Model file for the job. Use its own axes, mm. Face numbers are marked on the shaded views. A direction names the side the tool comes from. Coordinates: 2 decimals unless noted, no trailing zeros. Order: outer loops, then holes, each group sorted by start corner. A loop starts at its lowest first (then second) coordinate and runs counter-clockwise, first axis right, second up.
from build123d import *

# Parameters (mm, degrees)
SKETCH_1_R          = 3
EXTRUDE_2_DEPTH     = 50
EXTRUDE_3_DEPTH     = 8
CUT_EXTRUDE_1_DEPTH = 26
SKETCH_3_R          = 4.5
EXTRUDE_4_DEPTH     = 1


with BuildPart() as part:
    # Sketch 1 → Extrude 2 (new body)
    with BuildSketch(Plane(origin=(0, 0, 0), x_dir=(1, 0, 0), z_dir=(0, 1, 0))):
        with Locations(Location((0, 0, 0), (0, 0, 270))):
            Circle(SKETCH_1_R)
    extrude(amount=EXTRUDE_2_DEPTH)

    # Sketch 1_3 → Extrude 3 (add)
    with BuildSketch(Plane(origin=(0, 0, 0), x_dir=(1, 0, 0), z_dir=(0, 1, 0))):
        with BuildLine():
            Line((-1, 4), (-1, 2.828427125))
            ThreePointArc((-1, 2.828427125), (0, 3), (1, 2.828427125))
            Line((1, 2.828427125), (1, 4))
            Line((1, 4), (-1, 4))
        make_face()
    extrude(amount=EXTRUDE_3_DEPTH)

    # Sketch 2 → Cut-Extrude 1 (cut)
    with BuildSketch(Plane(origin=(0, 50, 0), x_dir=(1, 0, 0), z_dir=(0, 1, 0))):
        Polygon((-1.2, 1.149545417), (1.2, 1.149545417), (1.2, 2.749545417), (0, 4.828006386), (-1.2, 2.749545417), align=None)
    extrude(amount=-CUT_EXTRUDE_1_DEPTH, mode=Mode.SUBTRACT)

    # Sketch 3 → Extrude 4 (add)
    with BuildSketch(Plane.XZ):
        with Locations(Location((0, 0, 0), (0, 0, 270))):
            Circle(SKETCH_3_R)
    extrude(amount=EXTRUDE_4_DEPTH)


solid = part.part
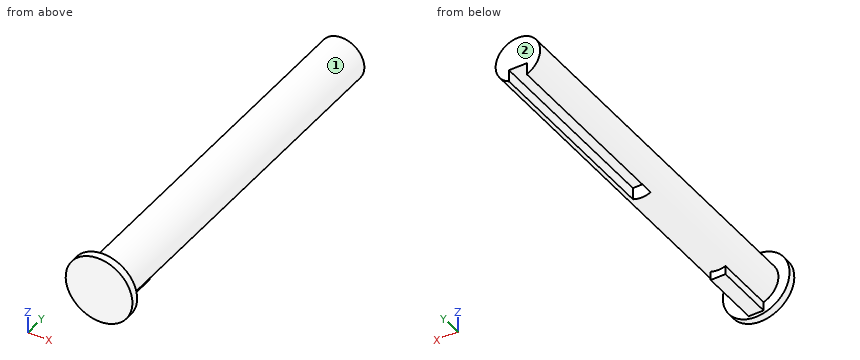
Q1. Probe line 1 (Y direction, x = 2.25, z = 3.5); line 2 (X direction, y = 4.5, z = -2.75); line 3 (Z direction, x = 0.25, y = 34.5). List the from-to ranges inside material, lowest first.
Established:
line 1: y = -1 to 0
line 2: x = -1.2 to 1.2
line 3: z = -1.15 to 2.99
Q2. Cut at B-B, the plane x = -1.75. List the corners of the cut face in (y, z).
Established:
outline: (-1, -4.15) - (0, -4.15) - (0, -2.44) - (50, -2.44) - (50, 2.44) - (0, 2.44) - (0, 4.15) - (-1, 4.15) - close
Q3. Cut at D-D, the plane z = -2. List the corners of the cut face in (x, y), plus the area to 3 significant figures.
Established:
outline: (-4.03, -1) - (4.03, -1) - (4.03, 0) - (2.24, 0) - (2.24, 50) - (1.2, 50) - (1.2, 24) - (-1.2, 24) - (-1.2, 50) - (-2.24, 50) - (-2.24, 0) - (-4.03, 0) - close
area: 169 mm2
Q4. Cut at A-A, the plane z = 0. List the corners of the cut face in (x, y), plus the area to 3 significant figures.
Established:
outline: (-4.5, -1) - (4.5, -1) - (4.5, 0) - (3, 0) - (3, 50) - (-3, 50) - (-3, 0) - (-4.5, 0) - close
area: 309 mm2
Q5. Cut at C-C, the plane y = 45.5. List the corners of the cut face in (x, z), plus the area to 3 significant figures.
Established:
outline: (-1.2, -2.75) - (-1.2, -1.15) - (1.2, -1.15) - (1.2, -2.75) arc R3 ccw (long way) to start
area: 24.0 mm2
Q6. Which spindle directions (+Z, -Z, +X, -X, +Y, -Y) get a long thin tool onto all of the face, cutting with end or side? Do the marked faces 1 and 2. Say none if no direction does.
Established:
face 1: +Y
face 2: +Z, -Z, +X, -X, +Y
Q7. Drop flat-ended pins along their axis: P1, Ø1.3, axis at y = 41.5, z = -1.5, coming from the +X side; P2, Ø0.6, axis at y = 4, z = -3.5, coming from the -X side; P3, Ø2, axis at x = -0.5, y = 4, coming from the -Z side. Give the stop position or say it passes through.
Established:
P1: stops at x = 2.88
P2: stops at x = -1
P3: stops at z = -4
